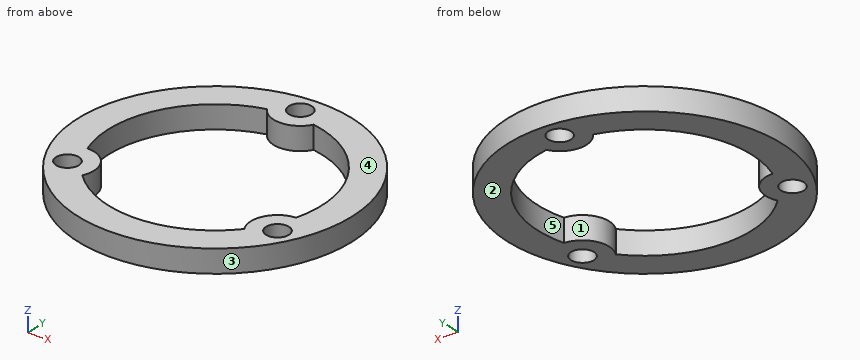
```python
from build123d import *

# Parameters (mm, degrees)
ESQUISSE1_R        = 18
ESQUISSE1_R_2      = 1.5
BOSS_EXTRU_2_DEPTH = 3


with BuildPart() as part:
    # Esquisse1 → Boss.-Extru.2 (new body)
    with BuildSketch(Plane.XY):
        Circle(ESQUISSE1_R)
        with Locations((-0.546712729, 15.490355231)):
            Circle(ESQUISSE1_R_2, mode=Mode.SUBTRACT)
        with Locations((-13.14168478, -8.218644727)):
            Circle(ESQUISSE1_R_2, mode=Mode.SUBTRACT)
        with Locations((13.688397508, -7.271710504)):
            Circle(ESQUISSE1_R_2, mode=Mode.SUBTRACT)
        with BuildLine():
            ThreePointArc((-3.468577117, 13.56351624), (-0.423261467, 11.992533082), (2.503723019, 13.774301109))
            ThreePointArc((2.503723019, 13.774301109), (11.869908833, 7.423292012), (13.480638187, -3.777882222))
            ThreePointArc((13.480638187, -3.777882222), (10.597469039, -5.629711358), (10.677033171, -9.055438293))
            ThreePointArc((10.677033171, -9.055438293), (0.493805045, -13.991288596), (-10.01206107, -9.785634018))
            ThreePointArc((-10.01206107, -9.785634018), (-10.174207571, -6.362821724), (-13.180756189, -4.718862816))
            ThreePointArc((-13.180756189, -4.718862816), (-12.363713879, 6.567996584), (-3.468577117, 13.56351624))
        make_face(mode=Mode.SUBTRACT)
    extrude(amount=BOSS_EXTRU_2_DEPTH)


solid = part.part
```
The listing builds one solid part. Answer for the finished solid, in the listing's coordinates (mm). Face numbers are marked on the shaded views. A direction names the side the tool comes from. Coordinates: 2 decimals unless noted, no trailing zeros. Write each loop counter-clockwise with the first axis right and the second up, starting at its lowest first coordinate (ties: lowest second). Pieces come first, ordered by that corner, then holes. Notation, with made-up numbers: (65, -30) - (88, -30) arc R19 ccw to (88, -22) - close; hole circle Ø2 at (43, 60). An arc over 180 degrees is marked (long way). One line per item, written item: value.
1) A tool of negligible diameter and unlimited length cuts with its end or side. For the marked faces 1 and 2, from which of +Z, -Z, +X, -X, +Y, -Y can it reach the whole face along a straight path? Write none if from no direction.
Geometry check:
face 1: +Z, -Z
face 2: -Z, +X, -X, +Y, -Y
2) Consider line 1 along X through (y, z) = (-7, 1.25); line 2 along Y through (x, z) = (-12, 1.4); line 3 along Y through (x, z) = (-7, 0.8). Determine where each line is inside the solid, lowest interval first. Write a range as from..to.
Geometry check:
line 1: x = -16.58..-14.02, -12.27..-9.86, 10.2..12.21, 15.16..16.58
line 2: y = -13.42..-9.19, -7.25..-4.91, 7.21..13.42
line 3: y = -16.58..-12.12, 12.12..16.58
3) Find section B-B (x = 14.5). Give the vertices of the cut face in (y, z), and give its area (3 significant figures).
Geometry check:
outline: (-10.67, 0) - (-8.53, 0) - (-8.53, 3) - (-10.67, 3) - close; (-6.01, 0) - (10.67, 0) - (10.67, 3) - (-6.01, 3) - close
area: 56.4 mm2
4) For a pull along X with two mould halves and no side action, classify the marked faces 3, 4 and 5 as pulls with the +X half, pulls with the -X half, needs draft (parallel to the pull), parting line crosses it, or undercut.
Geometry check:
face 3: parting line crosses it
face 4: needs draft
face 5: undercut
5) Find section A-A (y = 0). Give the vertices of the cut face in (x, z), and give its area (3 significant figures).
Geometry check:
outline: (-18, 0) - (-14, 0) - (-14, 3) - (-18, 3) - close; (14, 0) - (18, 0) - (18, 3) - (14, 3) - close
area: 24.0 mm2
6) Find section C-C (x = 0). Give the vertices of the cut face in (y, z).
Geometry check:
outline: (-18, 0) - (-14, 0) - (-14, 3) - (-18, 3) - close; (12.03, 0) - (14.09, 0) - (14.09, 3) - (12.03, 3) - close; (16.89, 0) - (18, 0) - (18, 3) - (16.89, 3) - close
7) Find section D-D (z = 1.85). Give the vertices of the cut face in (x, y), and give its area (3 significant figures).
Geometry check:
outline: circle Ø36 at (0, 0); hole circle Ø3 at (-13.14, -8.22); hole (-13.18, -4.72) arc R3.5 cw to (-10.01, -9.79) arc R14 ccw to (10.68, -9.06) arc R3.5 cw to (13.48, -3.78) arc R14 ccw to (2.5, 13.77) arc R3.5 cw to (-3.47, 13.56) arc R14 ccw to start; hole circle Ø3 at (-0.55, 15.49); hole circle Ø3 at (13.69, -7.27)
area: 406 mm2
